Here's how the part is built. I have some questions about the finished solid (model axes, mm). Coordinates: 2 decimals unless noted, no trailing zeros. Order: outer loops, then holes, each group sorted by start corner. A loop starts at its lowest first (then second) coordinate and runs counter-clockwise, first axis right, second up. Notation, with made-up numbers: (60, 12) -> (79, 12) arc R22 cw to (79, 20) -> close; hole circle Ø10 at (48, 11). An arc over 180 degrees is marked (long way). One line per item, written item: value. Start each with the question number.
```python
from build123d import *

# Parameters (mm, degrees)
SKETCH1_W      = 187.325
SKETCH1_H      = 174.625
SKETCH1_R      = 8.5328125
SKETCH1_R_2    = 47.625
EXTRUDE1_DEPTH = 6.35
FILLET1_R      = 6.35


with BuildPart() as part:
    # Sketch1 → Extrude1 (new body)
    with BuildSketch(Plane.XY):
        Rectangle(SKETCH1_W, SKETCH1_H)
        with Locations((-65.0875, 65.0875)):
            Circle(SKETCH1_R, mode=Mode.SUBTRACT)
        with Locations((65.0875, 65.0875)):
            Circle(SKETCH1_R, mode=Mode.SUBTRACT)
        with Locations((65.0875, -65.0875)):
            Circle(SKETCH1_R, mode=Mode.SUBTRACT)
        with Locations((-65.0875, -65.0875)):
            Circle(SKETCH1_R, mode=Mode.SUBTRACT)
        Circle(SKETCH1_R_2, mode=Mode.SUBTRACT)
    extrude(amount=EXTRUDE1_DEPTH)

    # Fillet1
    fillet1_edges = [part.edges().sort_by_distance(p)[0] for p in [
        (-93.6625, 87.3125, 3.175),
        (93.6625, 87.3125, 3.175),
        (93.6625, -87.3125, 3.175),
        (-93.6625, -87.3125, 3.175),
    ]]
    fillet(fillet1_edges, radius=FILLET1_R)


solid = part.part
```
Q1. Imagine slicing it at C-C (z = 4). Count the separate pieces of the cut face and the enclosed holes in it, plus the area to 3 significant figures.
Q2. I need wall thicknesses on line 1 (X direction, y = 65, z = 2.25); line 2 (X direction, y = -1, z = 3.25); line 3 (X direction, y = -69, z = 6). Which ranges of each line are inside material? Lowest first, please.
Q3. Imagine slicing it at D-D (y = -62). Write out the boundary of the cut face in (x, z), plus the area to 3 significant figures.
Q4. If we mould it in two halves opening along Y, with no side actions, what happens to faces 1 (the face through (-60.5, 72.28, 3.13)), 2 (the face through (91.753, -85.502, 3.219)), 3 (the face through (63.98, 73.55, 3.13)), 4 (the face through (-43, 21, 0))? For each: +Y half, -Y half, draft (parallel to the pull), parting line (faces both ways), or undercut.
Completed:
1. separate pieces: 1
1. enclosed holes: 5
1. area: 24,600 mm2
2. line 1: x = -93.66 to -73.62, -56.56 to 56.56, 73.62 to 93.66
2. line 2: x = -93.66 to -47.61, 47.61 to 93.66
2. line 3: x = -93.66 to -72.67, -57.5 to 57.5, 72.67 to 93.66
3. outline: (-93.66, 0) -> (-73.04, 0) -> (-73.04, 6.35) -> (-93.66, 6.35) -> close; (-57.13, 0) -> (57.13, 0) -> (57.13, 6.35) -> (-57.13, 6.35) -> close; (73.04, 0) -> (93.66, 0) -> (93.66, 6.35) -> (73.04, 6.35) -> close
3. area: 987 mm2
4. face 1: undercut
4. face 2: -Y half
4. face 3: undercut
4. face 4: draft
